The model under review builds one solid part; all positions refer to its coordinate system, in mm. Round coordinates to 2 decimals unless told otherwise and drop trailing zeros. Order: outer loops, then holes, each group sorted by start corner. A loop starts at its lowest first (then second) coordinate and runs counter-clockwise, first axis right, second up. Notation, with made-up numbers: M 20,25.5 L 53,25.5 A12 cw 53,41.5 Z; hole C 58,59.5 d8. An arc over 180 degrees is marked long. Answer as CSV lines item,"result". Start each with the question number.
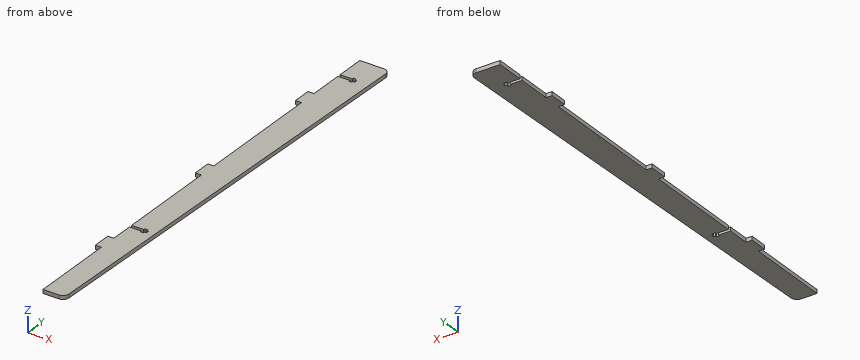
from build123d import *

# Parameters (mm, degrees)
BOSS_EXTRUDE1_DEPTH = 1.5875
SKETCH1_4_W         = 5
SKETCH1_4_H         = 15
BOSS_EXTRUDE2_DEPTH = 1.5875
SKETCH1_5_W         = 2.5
SKETCH1_5_H         = 5.2
SKETCH1_5_W_2       = 14
SKETCH1_5_H_2       = 2.6
CUT_EXTRUDE2_DEPTH  = 2.5875
LPATTERN1_COUNT     = 3
LPATTERN1_PITCH     = 120
LPATTERN3_COUNT     = 2
LPATTERN3_PITCH     = 250
FILLET1_R           = 5


with BuildPart() as part:
    # Sketch1 → Boss-Extrude1 (new body, symmetric)
    with BuildSketch(Plane.XY):
        Polygon((0, 0), (0, -380), (18, -380), (25, 0), align=None)
    extrude(amount=BOSS_EXTRUDE1_DEPTH, both=True)

    # Sketch1_4 → Boss-Extrude2 (add, symmetric)
    with BuildSketch(Plane.XY):
        with Locations((-2.5, -62.5)):
            Rectangle(SKETCH1_4_W, SKETCH1_4_H)
    boss_extrude2 = extrude(amount=BOSS_EXTRUDE2_DEPTH, both=True)

    # Sketch1_5 → Cut-Extrude2 (cut, symmetric)
    with BuildSketch(Plane.XY):
        with Locations((11.25, -25)):
            Rectangle(SKETCH1_5_W, SKETCH1_5_H)
        with Locations((7, -25)):
            Rectangle(SKETCH1_5_W_2, SKETCH1_5_H_2)
    cut_extrude2 = extrude(amount=CUT_EXTRUDE2_DEPTH, both=True, mode=Mode.SUBTRACT)

    # LPattern1: Boss-Extrude2 ×3
    with Locations(*[(0, -i * LPATTERN1_PITCH, 0) for i in range(1, LPATTERN1_COUNT)]):
        add(boss_extrude2)

    # LPattern3: Cut-Extrude2 ×2
    with Locations(*[(0, -i * LPATTERN3_PITCH, 0) for i in range(1, LPATTERN3_COUNT)]):
        add(cut_extrude2, mode=Mode.SUBTRACT)

    # Fillet1
    fillet1_edges = [part.edges().sort_by_distance(p)[0] for p in [
        (18, -380, 0),
        (25, 0, 0),
    ]]
    fillet(fillet1_edges, radius=FILLET1_R)


solid = part.part
Item 1: Wall thickness on probe 1 along Y at (x, z) = (0.5, 0.1); probe 2 along Y at (x, z) = (11.5, -1); probe 3 along Y at (x, z) = (16, 1.25): over which ranges is each line inside the solid? List them lowest first. Write a range as [from, to].
Item 2: For pin 1 (1 mm diameter, centred on x = -1.5, z = -1, fed in from +Y); pin 2 (1 mm diameter, centred on y = -276.5, z = -0.5, fed in from -X); pin 3 (0.8 mm diameter, centred on y = -274.5, z = 0.5, fed in from -X); pin 4 (1.5 mm diameter, centred on x = 21.5, y = -323, fed in from -Z), all flat-tipped, find the tip position at first contact; note any pin that passes through.
Item 3: Consider section A-A (y = -250). State the section outline as (x, z) points.
Item 4: Consider section B-B (y = -110.5). State the section outline as (x, z) points.
Reported:
1,probe 1,"y = [-380, -276.3], [-273.7, -26.3], [-23.7, 0]"
1,probe 2,"y = [-380, -277.6], [-272.4, -27.6], [-22.4, 0]"
1,probe 3,"y = [-379.07, 0]"
2,pin 1,"stops at y = -55"
2,pin 2,"stops at x = 0"
2,pin 3,"stops at x = 14"
2,pin 4,"passes through"
3,outline,"M 0,-1.59 L 20.39,-1.59 L 20.39,1.59 L 0,1.59 Z"
4,outline,"M 0,-1.59 L 22.96,-1.59 L 22.96,1.59 L 0,1.59 Z"
